Geometry: final body of the model. Coordinates: model frame, mm. A direction names the side the tool comes from. Give positions to 0.01 mm unless a question says otherwise; leave off trailing zeros. Write each loop counter-clockwise with the first axis right and the second up, starting at its lowest first coordinate (ties: lowest second). Pieces come first, ordered by that corner, then holes.
Q1. Section C-C (x = 116). Return the cut outline in (y, z).
Q2. Reachability of faces 4 (the flat face through (-41.86, 17.8, 64.09)), 5 (the flat face through (61.5, -0.2, 0)) from +Z, -Z, +X, -X, +Y, -Y: full face, straight path, thin tool, end or side. Return the list, or none.
Q3. Mould query, pull axis X, two halves, no side actions, for faces 1 (the flat face through (61.5, -0.2, 130)), 2 (the flat face through (60, 0, 64)), 3 (the flat face through (-41.93, 16.46, 64.09)). Classes: +X half, -X half, draft (parallel to the pull), parting line (faces both ways), or undercut.
Q4. Section A-A (z = 56.5). Return the cut outline in (x, y).
Q5. Section D-D (x = -34). Return the cut outline in (y, z), plus the area to 3 significant figures.
Q6. Pin query (flat end, axial travel): pin 1 Ø8 at (y, z) = (20, 65.5) entering from -X; pin 2 Ø2 at (y, z) = (14, 25) entering from -X; pin 3 Ø1 at (y, z) = (5.5, 25.5) entering from -X. Return the tip coordinate at first contact, or that it passes through.
Q7. Line query: line 1 (X direction, y = -0.4, z = 110); line 2 (Y direction, x = -10.5, z = 12.5); line 3 (X direction, y = -0.2, z = 110). Output: solid intervals per line, ascending.
Q8. Section B-B (y = 31.5). Return the cut outline in (x, z), plus the area to 3 significant figures.
from build123d import *

# Parameters (mm, degrees)
EXTRU_MINCE1_DEPTH = 130
D_GAGEMENT_M32_D   = 3.4


with BuildPart() as part:
    # Esquisse2 → Extru.-Mince1 (new body)
    with BuildSketch(Plane.XY):
        Polygon((-59.170699115, 35.114), (-24.057682042, 0), (145.942317958, 0), (181.056317958, 35.113017073), (181.763414842, 34.405900395), (146.356523321, -1), (-24.471903803, -1), (-59.877815794, 34.406903116), align=None)
    extrude(amount=EXTRU_MINCE1_DEPTH)

    # Dégagement M32 (through all)
    with Locations(Plane(origin=(0, 0, 0), x_dir=(-1, 0, 0), z_dir=(0, 1, 0))):
        with Locations((18.357682042, 20), (-140.242317958, 20), (-140.242317958, 110), (18.357682042, 110)):
            Hole(D_GAGEMENT_M32_D / 2)


solid = part.part
Computed:
1. outline: (-1, 0) - (0, 0) - (0, 130) - (-1, 130) - close
2. face 4: +Z, -Z, +Y
2. face 5: -Z, +X, -X, +Y, -Y
3. face 1: draft
3. face 2: undercut
3. face 3: -X half
4. outline: (-59.88, 34.41) - (-24.47, -1) - (146.36, -1) - (181.76, 34.41) - (181.06, 35.11) - (145.94, 0) - (-24.06, 0) - (-59.17, 35.11) - close
5. outline: (8.53, 0) - (9.94, 0) - (9.94, 130) - (8.53, 130) - close
5. area: 184 mm2
6. pin 1: stops at x = -49.47
6. pin 2: stops at x = -40.47
6. pin 3: stops at x = -31.47
7. line 1: x = -25.07 to -20.06, -16.66 to 138.54, 141.94 to 146.96
7. line 2: y = -1 to 0
7. line 3: x = -25.27 to -20.06, -16.66 to 138.54, 141.94 to 147.16
8. outline: (-56.97, 0) - (-55.56, 0) - (-55.56, 130) - (-56.97, 130) - close; (177.44, 0) - (178.86, 0) - (178.86, 130) - (177.44, 130) - close
8. area: 368 mm2
